Design review of the part built by this model. Coordinates are the model's own, in mm. Face numbers are marked on the shaded views. A direction names the side the tool comes from. Round coordinates to 2 decimals unless told otherwise and drop trailing zeros. Loops run counter-clockwise (first coordinate to the right, second up) from the corner with the lowest first, then second, coordinate; pieces in that order, holes last. Notation, with made-up numbers: (-11, -22.75) - (45, -22.75) arc R26 cw to (45, 13.25) - close; hole circle Ø8 at (-25, 39.5). An arc over 180 degrees is marked (long way). Answer as CSV lines item,"result". Start each with the question number.
(1) Consider section A-A (x = -34). Give the boundary of the cut face in (y, z), and give its area (3 significant figures).
(2) Consider section D-D (x = -108). Give the boundary of the cut face in (y, z).
(3) Consider section B-B (z = -16.5). Give the boundary of the cut face in (x, y), and give its area (3 significant figures).
(4) Mouldability with a two-part tool opening along Z and no side actions: class the marked faces 4, 5 and 6 as released by +Z, released by -Z, zero draft, split by the parting line, or undercut.
(5) Consider section C-C (z = -5). Give the boundary of the cut face in (x, y) (3 decimals).
(6) For the marked faces 1, 2 and 3, list the 3-axis set-ups (+Z, -Z, +X, -X, +Y, -Y) from which the entire face can be reached by the end or side of a thin tool; tool diameter is ignored.
(7) Wall thickness on L1, parallel to Z at x = -32, y = 36.5; L2, parallel to X at y = 27, z = -20.5; L3, parallel to X at y = 29, z = 13: over which ranges is each line inside the solid? List them lowest first.
(8) For P1, Ø10, axis at x = -35, y = 25.5, coming from the +Z side; P2, Ø2, axis at y = 13, z = 0, coming from the -X side; P3, Ø3, axis at x = -116.5, z = 21.5, coming from the +Y side (3 decimals), all flat-tipped, find the tip position at first contact; note any pin that passes through.
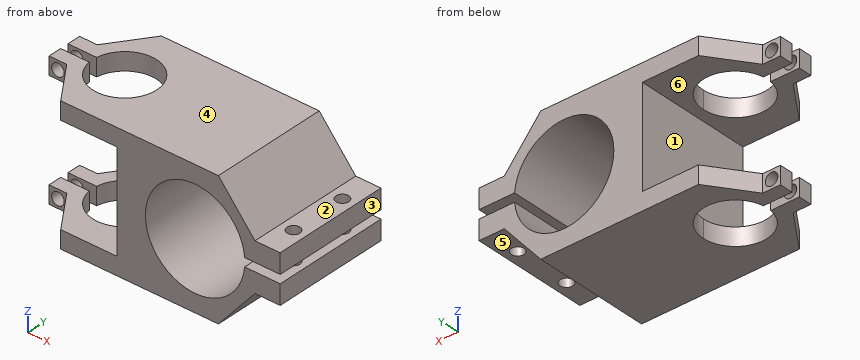
from build123d import *

# Parameters (mm, degrees)
BOSS_EXTRUDE1_DEPTH = 41.91
SKETCH2_R           = 11.43
CUT_EXTRUDE1_DEPTH  = 56.388
SKETCH3_W           = 21.064654828
SKETCH3_H           = 1.524
CUT_EXTRUDE3_DEPTH  = 56.388
SKETCH4_R           = 2.2499955
CUT_EXTRUDE4_DEPTH  = 56.388
SKETCH5_R           = 2.286
CUT_EXTRUDE5_DEPTH  = 56.388


with BuildPart() as part:
    # Sketch1 → Boss-Extrude1 (new body)
    with BuildSketch(Plane(origin=(0, 0, 0), x_dir=(1, 0, 0), z_dir=(0, 1, 0))):
        with BuildLine():
            Line((-121.13336204, 24.13), (-48.027058794, 24.13))
            Line((-48.027058794, 24.13), (-34.965614565, 8.563976916))
            Line((-34.965614565, 8.563976916), (-25.948796733, 8.563976916))
            Line((-25.948796733, 8.563976916), (-25.948796733, 1.524))
            Line((-25.948796733, 1.524), (-38.648796733, 1.524))
            ThreePointArc((-38.648796733, 1.524), (-74.14336204, 0), (-38.648796733, -1.524))
            Line((-38.648796733, -1.524), (-25.948796733, -1.524))
            Line((-25.948796733, -1.524), (-25.948796733, -8.563976916))
            Line((-25.948796733, -8.563976916), (-34.965614565, -8.563976916))
            Line((-34.965614565, -8.563976916), (-48.027058794, -24.13))
            Line((-48.027058794, -24.13), (-121.13336204, -24.13))
            Line((-121.13336204, -24.13), (-121.13336204, -17.78))
            Line((-121.13336204, -17.78), (-84.30336204, -17.78))
            Line((-84.30336204, -17.78), (-84.30336204, 17.78))
            Line((-84.30336204, 17.78), (-121.13336204, 17.78))
            Line((-121.13336204, 17.78), (-121.13336204, 24.13))
        make_face()
    extrude(amount=BOSS_EXTRUDE1_DEPTH)

    # Sketch2 → Cut-Extrude1 (cut)
    with BuildSketch(Plane.XY.offset(24.13)):
        with Locations((-99.54336204, 20.955)):
            Circle(SKETCH2_R)
    extrude(amount=-CUT_EXTRUDE1_DEPTH, mode=Mode.SUBTRACT)

    # Sketch3 → Cut-Extrude3 (cut)
    with BuildSketch(Plane.XY.offset(24.13)):
        Polygon((-121.13336204, 14.605), (-114.78336204, 14.605), (-104.400968543, 0), (-121.13336204, 0), align=None)
        Polygon((-104.400968543, 41.91), (-121.13336204, 41.91), (-121.13336204, 27.305), (-114.78336204, 27.305), align=None)
        with Locations((-110.601034626, 20.193)):
            Rectangle(SKETCH3_W, SKETCH3_H)
        with Locations((-110.601034626, 21.717)):
            Rectangle(SKETCH3_W, SKETCH3_H)
    extrude(amount=-CUT_EXTRUDE3_DEPTH, mode=Mode.SUBTRACT)

    # Sketch4 → Cut-Extrude4 (cut)
    with BuildSketch(Plane(origin=(0, 27.305, 0), x_dir=(1, 0, 0), z_dir=(0, 1, 0))):
        with Locations(Location((-117.95836204, 20.955, 0), (0, 0, 180))):
            Circle(SKETCH4_R)
        with Locations(Location((-117.95836204, -20.955, 0), (0, 0, 180))):
            Circle(SKETCH4_R)
    extrude(amount=-CUT_EXTRUDE4_DEPTH, mode=Mode.SUBTRACT)

    # Sketch5 → Cut-Extrude5 (cut)
    with BuildSketch(Plane.XY.offset(8.563976916)):
        with Locations((-30.457205649, 31.115)):
            Circle(SKETCH5_R)
        with Locations((-30.457205649, 10.795)):
            Circle(SKETCH5_R)
    extrude(amount=-CUT_EXTRUDE5_DEPTH, mode=Mode.SUBTRACT)


solid = part.part
Determined:
1,outline,"(0, -8.56) - (41.91, -8.56) - (41.91, -1.52) - (0, -1.52) - close; (0, 1.52) - (41.91, 1.52) - (41.91, 8.56) - (0, 8.56) - close"
1,area,"590 mm^2"
2,outline,"(5.06, -24.13) - (13.27, -24.13) - (13.27, -17.78) - (5.06, -17.78) - close; (5.06, 17.78) - (13.27, 17.78) - (13.27, 24.13) - (5.06, 24.13) - close; (28.64, -24.13) - (36.85, -24.13) - (36.85, -17.78) - (28.64, -17.78) - close; (28.64, 17.78) - (36.85, 17.78) - (36.85, 24.13) - (28.64, 24.13) - close"
3,outline,"(-84.3, 0) - (-62.99, 0) - (-62.99, 41.91) - (-84.3, 41.91) - close; (-49.74, 0) - (-41.62, 0) - (-41.62, 41.91) - (-49.74, 41.91) - close"
3,area,"1,230 mm^2"
4,face 4,"released by +Z"
4,face 5,"released by -Z"
4,face 6,"undercut"
5,outline,"(-84.303, 0) - (-73.426, 0) - (-73.426, 41.91) - (-84.303, 41.91) - close; (-39.301, 0) - (-25.949, 0) - (-25.949, 41.91) - (-39.301, 41.91) - close; hole circle Ø4.572 at (-30.457, 10.795); hole circle Ø4.572 at (-30.457, 31.115)"
6,face 1,"-X, +Y, -Y"
6,face 2,"+Z, +X, +Y, -Y"
6,face 3,"+Z, -Z, +X, +Y, -Y"
7,L1,"z = -8.56 to -1.52, 1.52 to 8.56"
7,L2,"x = -121.13 to -120.16, -115.75 to -109.24, -89.84 to -44.98"
7,L3,"x = -84.3 to -68.49, -44.23 to -38.69"
8,P1,"stops at z = 14.56"
8,P2,"stops at x = -84.3"
8,P3,"stops at y = 27.305"
